```python
from build123d import *

# Parameters (mm, degrees)
CUT_EXTRUDE1_START = 15
CUT_EXTRUDE1_DEPTH = 2
CUT_EXTRUDE2_START = 15.5
CUT_EXTRUDE2_DEPTH = 25
SKETCH5_R          = 3
CUT_EXTRUDE3_DEPTH = 31
SKETCH9_R          = 3
CUT_EXTRUDE4_DEPTH = 6
CUT_EXTRUDE4_DRAFT = -8


with BuildPart() as part:
    # Sketch1 → Revolve1 (revolve)
    with BuildSketch(Plane.XY, mode=Mode.PRIVATE) as revolve1_sk:
        Polygon((-98.694744318, 0), (87.305255682, 0), (87.305255682, 16.922649731), (86.305255682, 17.5), (70.305255682, 17.5), (70.305255682, 19), (21.305255682, 19), (21.305255682, 22.5), (-0.694744318, 22.5), (-0.694744318, 17.5), (-36.694744318, 17.5), (-38.694744318, 17.147346039), (-38.694744318, 15), (-97.694744318, 15), (-98.694744318, 14.422649731), align=None)
    revolve(revolve1_sk.sketch.rotate(Axis((-98.694744318, 0, 0), (1, 0, 0)), 180), axis=Axis((-98.694744318, 0, 0), (1, 0, 0)))

    # Sketch2 → Cut-Extrude1 (cut)
    with BuildSketch(Plane.XY.offset(CUT_EXTRUDE1_START)):
        with BuildLine():
            Line((-89.694994324, 4.05), (-47.694994324, 4.05))
            ThreePointArc((-47.694994324, 4.05), (-43.694994324, 0.05), (-47.694994324, -3.95))
            Line((-47.694994324, -3.95), (-89.694994324, -3.95))
            ThreePointArc((-89.694994324, -3.95), (-93.694994324, 0.05), (-89.694994324, 4.05))
        make_face()
    extrude(amount=-CUT_EXTRUDE1_DEPTH, mode=Mode.SUBTRACT)

    # Sketch3 → Cut-Extrude2 (cut)
    with BuildSketch(Plane.XY.offset(CUT_EXTRUDE2_START)):
        with BuildLine():
            Line((27.305255682, 4), (69.305255682, 4))
            ThreePointArc((69.305255682, 4), (74.305255682, -1), (69.305255682, -6))
            Line((69.305255682, -6), (27.305255682, -6))
            ThreePointArc((27.305255682, -6), (22.305255682, -1), (27.305255682, 4))
        make_face()
    extrude(amount=CUT_EXTRUDE2_DEPTH, mode=Mode.SUBTRACT)

    # Sketch5 → Cut-Extrude3 (cut)
    with BuildSketch(Plane.ZY.offset(98.694744318)):
        Circle(SKETCH5_R)
    extrude(amount=-CUT_EXTRUDE3_DEPTH, mode=Mode.SUBTRACT)


with BuildPart() as cut_extrude4_tool:
    # Sketch9 → Cut-Extrude4 (with draft: the straight prism first)
    with BuildSketch(Plane(origin=(87.305255682, 0, 0), x_dir=(0, 0, -1), z_dir=(1, 0, 0))):
        with Locations(Location((0, 0, 0), (0, 0, 180))):
            Circle(SKETCH9_R)
    extrude(amount=-CUT_EXTRUDE4_DEPTH)
    # Cut-Extrude4: the draft: its side faces are tilted about the plane it starts from
    cut_extrude4_sides = [cut_extrude4_tool.faces().sort_by_distance(p)[0] for p in [
        (84.305255682, 0, -3),
    ]]
    draft(cut_extrude4_sides, Plane(origin=(87.305255682, 0, 0), x_dir=(0, 0, -1), z_dir=(1, 0, 0)), CUT_EXTRUDE4_DRAFT)


with BuildPart() as part_1:
    add(part.part)

    # Cut-Extrude4: cut by cut_extrude4_tool
    add(cut_extrude4_tool.part, mode=Mode.SUBTRACT)


solid = part_1.part
```
Geometry check sheet. Reference: the model listing, model coordinates, mm. A direction names the side the tool comes from. Coordinates: 2 decimals unless noted, no trailing zeros. Write each loop counter-clockwise with the first axis right and the second up, starting at its lowest first coordinate (ties: lowest second). Pieces come first, ordered by that corner, then holes. Notation, with made-up numbers: M -2.75,40.25 L 22.25,40.25 A9 ccw 22.25,47.25 Z; hole C 79.5,-24 d9. An arc over 180 degrees is marked long. Use one line per item in the form item = value. Start each with the question number.
1) Section check C-C on x = -24.5. Enter the section's corners in (y, z), and give its area (3 significant figures).
2) Section check D-D on x = 42. Enter the section's corners in (y, z).
3) Section check B-B on x = -80. Enter the section's corners in (y, z), and give its area (3 significant figures).
4) Thickness scan on probe 1 along X at (y, z) = (-19.5, 2.5); probe 2 along X at (y, z) = (-15, -6); probe 3 along Z at (x, y) = (-56, -0.5). Record the ranges inside material, lowest first. Write a range as from..to.
5) Set-up check for faces 1 (the cylindrical face through (-93.694, -0.038, 13.792)), 2 (the flat face through (81.305, 0, 0)), 3 (the cylindrical face through (-83, 0, -3)), 4 (the flat face through (-98.695, 3.4, -0.2)): record each of +Z, -Z, +X, -X, +Y, -Y from which the full face is reachable in a straight line by a thin tool's end or side.
6) Release check for a two-part mould opening along Y. For faces 5 (the cylindrical face through (45.462, -8.767, 16.856)), 6 (the flat face through (48, 4, 17)), 7 (the flat face through (-38.695, 0.1, 15.2)) record: pulls with the +Y half, pulls with the -Y half, needs draft (parallel to the pull), parting line crosses it, or undercut.
7) Go/stop test with flat-tipped pins: pin 1 Ø6.5 at (x, y) = (-61.5, 0) entering from +Z; pin 2 Ø1 at (x, z) = (8, 3.5) entering from -Y; pin 3 Ø10 at (x, y) = (-25, 9.5) entering from -Z. Record where each tip stops, or that it passes through.
Responses:
q1.outline = C 0,0 d35
q1.area = 962 mm2
q2.outline = M -6,15.5 L -6,18.03 A19 ccw long 4,18.57 L 4,15.5 Z
q3.outline = M -3.95,13 L -3.95,14.47 A15 ccw long 4.05,14.44 L 4.05,13 Z; hole C 0,0 d6
q3.area = 664 mm2
q4.probe_1 = -0.69..21.31
q4.probe_2 = -38.69..87.31
q4.probe_3 = -14.99..13
q5.face_1 = +Z
q5.face_2 = +X
q5.face_3 = -X
q5.face_4 = +Z, -Z, -X, +Y, -Y
q6.face_5 = parting line crosses it
q6.face_6 = undercut
q6.face_7 = needs draft
q7.pin_1 = 13
q7.pin_2 = -22.3
q7.pin_3 = -16.91
